```python
from build123d import *

# Parameters (mm, degrees)
F0_W     = 50
F0_H     = 10
F0_R     = 2.5
F1_DEPTH = 5
F2_DEPTH = 2


with BuildPart() as f1:
    # F0 (on Right) → F1 (new body)
    with BuildSketch(Plane.YZ):
        with Locations((-25, 5)):
            Rectangle(F0_W, F0_H)
        with Locations((-38.6293791234, 5)):
            Circle(F0_R, mode=Mode.SUBTRACT)
        with Locations((-8.6293791234, 5)):
            Circle(F0_R, mode=Mode.SUBTRACT)
    extrude(amount=F1_DEPTH)

    # F2 (cut): a face of the model
    f2_faces = [f1.faces().sort_by_distance(p)[0] for p in [
        (5, -25.1168236174, 5),
    ]]
    extrude(f2_faces, amount=-F2_DEPTH, mode=Mode.SUBTRACT)


solid = f1.part
```
Source: CAD feature listing. Evaluate the final solid. Frame: model axes, mm. Round coordinates to 2 decimals unless told otherwise and drop trailing zeros. Loops run counter-clockwise (first coordinate to the right, second up) from the corner with the lowest first, then second, coordinate; pieces in that order, holes last. Notation, with made-up numbers: M 44.25,33 L 79.25,33 A22 cw 79.25,69 Z; hole C 89,-24 d5. An arc over 180 degrees is marked long. Use a Markdown table: item, result. Add a question column.
1. Line query: line 1 (Y direction, x = 0.9, z = 6); line 2 (Y direction, x = 0.9, z = 5.25); line 3 (Z direction, x = 1.25, y = -39). Output: solid intervals per line, ascending.
2. Contact query for flat-ended pins moving along their axis: P1, Ø1, axis at x = 1, y = -35.5, coming from the -Z side; P2, Ø4.5, axis at y = -38.63, z = 5, coming from the -X side. Output: stop coordinate, or through.
3. Section query B-B on y = -40. Return the cut outline in (x, z), then the cut area to 3 significant figures.
4. Section query C-C on x = 1.95. Return the cut outline in (y, z), then the cut area to 3 significant figures.
5. Section query A-A on z = 5. Return the cut outline in (x, y).
6. Mould query, pull axis Y, two halves, no side actions, for faces 1 (the flat face through (1, -50, 5)), 2 (the cylindrical face through (1.479, -41.127, 5.11)), 3 (the flat face through (3, -25, 5)), 4 (the cylindrical face through (1.479, -6.245, 5.751)). Classes: pulls with the +Y half, pulls with the -Y half, needs draft (parallel to the pull), parting line crosses it, or undercut.
7. Section query D-D on z = 3. Return the cut outline in (x, y).
Reported:
| question | item | result |
|---|---|---|
| 1 | line 1 | y = -50 to -40.92, -36.34 to -10.92, -6.34 to 0 |
| 1 | line 2 | y = -50 to -41.12, -36.14 to -11.12, -6.14 to 0 |
| 1 | line 3 | z = 0 to 2.53, 7.47 to 10 |
| 2 | P1 | stops at z = 0 |
| 2 | P2 | passes through |
| 3 | outline | M 0,0 L 3,0 L 3,2.91 L 0,2.91 Z; M 0,7.09 L 3,7.09 L 3,10 L 0,10 Z |
| 3 | area | 17.5 mm² |
| 4 | outline | M -50,0 L 0,0 L 0,10 L -50,10 Z; hole C -38.63,5 d5; hole C -8.63,5 d5 |
| 4 | area | 461 mm² |
| 5 | outline | M 0,-50 L 3,-50 L 3,-41.13 L 0,-41.13 Z; M 0,-36.13 L 3,-36.13 L 3,-11.13 L 0,-11.13 Z; M 0,-6.13 L 3,-6.13 L 3,0 L 0,0 Z |
| 6 | face 1 | pulls with the -Y half |
| 6 | face 2 | undercut |
| 6 | face 3 | needs draft |
| 6 | face 4 | undercut |
| 7 | outline | M 0,-50 L 3,-50 L 3,-40.13 L 0,-40.13 Z; M 0,-37.13 L 3,-37.13 L 3,-10.13 L 0,-10.13 Z; M 0,-7.13 L 3,-7.13 L 3,0 L 0,0 Z |
